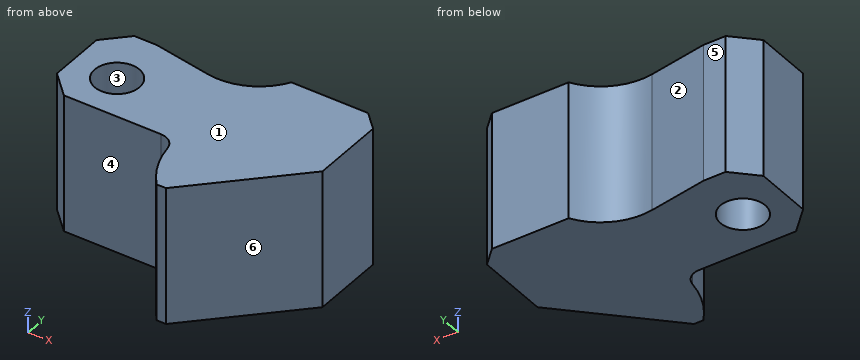
```python
from build123d import *

# Parameters (mm, degrees)
SKETCH1_R           = 7
BOSS_EXTRUDE2_DEPTH = 43


with BuildPart() as part:
    # Sketch1 → Boss-Extrude2 (new body)
    with BuildSketch(Plane.XY):
        with BuildLine():
            Line((0, 0), (7, 7))
            Line((7, 7), (14, 7))
            Line((14, 7), (32.243084988, 3.783251905))
            ThreePointArc((32.243084988, 3.783251905), (43.574972961, 5.276069151), (52, 13))
            Line((52, 13), (76, 13))
            Line((76, 13), (81, 8))
            Line((81, 8), (81, -15))
            Line((81, -15), (52, -44))
            Line((52, -44), (49.0910977, -44))
            ThreePointArc((49.0910977, -44), (44.652125503, -37.115672061), (42.3152953, -29.264705882))
            ThreePointArc((42.3152953, -29.264705882), (40.634892339, -26.213413768), (37.369656558, -25))
            Line((37.369656558, -25), (7, -25))
            Line((7, -25), (0, -18))
            Line((0, -18), (0, 0))
        make_face()
        with Locations((14, -11)):
            Circle(SKETCH1_R, mode=Mode.SUBTRACT)
    extrude(amount=BOSS_EXTRUDE2_DEPTH)


solid = part.part
```
Source: CAD feature listing. Evaluate the final solid. Frame: model axes, mm. Face numbers are marked on the shaded views. A direction names the side the tool comes from. Coordinates: 2 decimals unless noted, no trailing zeros. Loops run counter-clockwise (first coordinate to the right, second up) from the corner with the lowest first, then second, coordinate; pieces in that order, holes last. Notation, with made-up numbers: (71, -18) -> (108, -18) arc R14 ccw to (108, 2) -> close; hole circle Ø10 at (46, -15). An arc over 180 degrees is marked (long way). One line per item, written item: value. Start each with the question number.
Q1. Contact query for flat-ended pins moving along their axis: P1, Ø6, axis at y = -34, z = 27, coming from the -X side; P2, Ø8, axis at y = -27, z = 31.5, coming from the +X side; P3, Ø5.5, axis at x = 12, z = 26.5, coming from the +Y side; P4, Ø3, axis at y = 1, z = 11.5, coming from the -X side. Output: stop coordinate, or through.
Q2. Section query D-D, the plane y = 2. Return the cut outline in (x, z).
Q3. Section query B-B, the plane z = 33. Return the cut outline in (x, y).
Q4. Set-up query: the marked faces 4, 5 and 6. Return all of +Z, -Z, +X, -X, +Y, -Y with unobstructed straight access to the full face (end or side cutting, diameter ignored); none if empty.
Q5. Section query A-A, the plane y = -11. Return the cut outline in (x, z), and give its area (3 significant figures).
Q6. Section query C-C, the plane x = 12.5. Return the cut outline in (y, z).
Q7. Line query: line 1 along Y through (x, z) = (14, 27); line 2 along Y through (x, z) = (71, 24.5); line 3 along Y through (x, z) = (11, 38). Output: solid intervals per line, ascending.
Q8. Mould query, pull axis Y, two halves, no side actions, for the marked faces 1, 2 and 3. Classes: pulls with the +Y half, pulls with the -Y half, needs draft (parallel to the pull), parting line crosses it, or undercut.
Results:
1. P1: x = 42.63
1. P2: x = 73
1. P3: y = 7
1. P4: x = 0
2. outline: (2, 0) -> (81, 0) -> (81, 43) -> (2, 43) -> close
3. outline: (0, -18) -> (7, -25) -> (37.37, -25) arc R5 cw to (42.32, -29.26) arc R29 ccw to (49.09, -44) -> (52, -44) -> (81, -15) -> (81, 8) -> (76, 13) -> (52, 13) arc R19 cw to (32.24, 3.78) -> (14, 7) -> (7, 7) -> (0, 0) -> close; hole circle Ø14 at (14, -11)
4. face 4: +Z, -Z, -X, -Y
4. face 5: +Z, -Z, -X, +Y
4. face 6: +Z, -Z, +X, -Y
5. outline: (0, 0) -> (7, 0) -> (7, 43) -> (0, 43) -> close; (21, 0) -> (81, 0) -> (81, 43) -> (21, 43) -> close
5. area: 2,880 mm^2
6. outline: (-25, 0) -> (-17.84, 0) -> (-17.84, 43) -> (-25, 43) -> close; (-4.16, 0) -> (7, 0) -> (7, 43) -> (-4.16, 43) -> close
7. line 1: -25 to -18, -4 to 7
7. line 2: -25 to 13
7. line 3: -25 to -17.32, -4.68 to 7
8. face 1: needs draft
8. face 2: pulls with the +Y half
8. face 3: undercut
